```python
from build123d import *

# Parameters (mm, degrees)
BOSS_EXTRUDE1_DEPTH     = 114.3
CUT_EXTRUDE1_DEPTH      = 116.702506455
CUT_EXTRUDE1_DEPTH_BACK = 116.702506455
SKETCH5_R               = 0.55245


with BuildPart() as part:
    # Sketch4 → Boss-Extrude1 (new, symmetric)
    with BuildSketch(Plane.XY):
        with BuildLine():
            Line((4.190365, -12.7), (10.11729625, -12.7))
            ThreePointArc((10.11729625, -12.7), (11.943543585, -11.943543585), (12.7, -10.11729625))
            Line((12.7, -10.11729625), (12.7, -4.190365))
            ThreePointArc((12.7, -4.190365), (12.42492494, -3.52627506), (11.760835, -3.2512))
            Line((11.760835, -3.2512), (11.429365, -3.2512))
            ThreePointArc((11.429365, -3.2512), (10.76527506, -3.52627506), (10.4902, -4.190365))
            Line((10.4902, -4.190365), (10.4902, -6.348478019))
            ThreePointArc((10.4902, -6.348478019), (9.830707141, -7.335478831), (8.666460301, -7.103895736))
            Line((8.666460301, -7.103895736), (5.299899128, -3.737334563))
            ThreePointArc((5.299899128, -3.737334563), (4.817571085, -3.015479634), (4.6482, -2.16399369))
            Line((4.6482, -2.16399369), (4.6482, 0))
            Line((4.6482, 0), (2.6035, 0))
            ThreePointArc((2.6035, 0), (1.840952505, -1.840952505), (0, -2.6035))
            Line((0, -2.6035), (0, -4.6482))
            Line((0, -4.6482), (2.16399369, -4.6482))
            ThreePointArc((2.16399369, -4.6482), (3.015479634, -4.817571085), (3.737334563, -5.299899128))
            Line((3.737334563, -5.299899128), (7.103895736, -8.666460301))
            ThreePointArc((7.103895736, -8.666460301), (7.335478831, -9.830707141), (6.348478019, -10.4902))
            Line((6.348478019, -10.4902), (4.190365, -10.4902))
            ThreePointArc((4.190365, -10.4902), (3.52627506, -10.76527506), (3.2512, -11.429365))
            Line((3.2512, -11.429365), (3.2512, -11.760835))
            ThreePointArc((3.2512, -11.760835), (3.52627506, -12.42492494), (4.190365, -12.7))
        make_face()
    extrude(amount=BOSS_EXTRUDE1_DEPTH, both=True)

    # Sketch5 → Cut-Extrude1 (cut, two sides: drawn at the far end of the back side and taken through both)
    with BuildSketch(Plane.XY.offset(-CUT_EXTRUDE1_DEPTH_BACK)):
        with Locations((10.356153152, -12.7)):
            Circle(SKETCH5_R)
        with Locations((5.796028019, -12.7)):
            Circle(SKETCH5_R)
        with Locations((12.7, -10.356153152)):
            Circle(SKETCH5_R)
        with Locations((12.7, -5.796028019)):
            Circle(SKETCH5_R)
    extrude(amount=CUT_EXTRUDE1_DEPTH + CUT_EXTRUDE1_DEPTH_BACK, mode=Mode.SUBTRACT)

    # Mirror1: part across plane


with BuildPart() as part_1:
    add(part.part)
    add(part.part.mirror(Plane(origin=(0, 0, 0), x_dir=(0, 0, 1), z_dir=(1, 0, 0))))

    # Mirror2: part across plane


with BuildPart() as part_2:
    add(part_1.part)
    add(part_1.part.mirror(Plane.ZX))


solid = part_2.part
```
The listing builds one solid part. Answer for the finished solid, in the listing's coordinates (mm). A direction names the side the tool comes from. Round coordinates to 2 decimals unless told otherwise and drop trailing zeros. Put each result on its own line as item: value. Start each with the question number.
(1) Given P1, Ø5, axis at y = -0.5, z = 48.5, coming from the -X side; P2, Ø3.5, axis at x = 0, z = -49.5, coming from the +Y side; P3, Ø1, axis at y = 2, z = -50.5, coming from the +X side, each flat-ended and moving along its own axis, determine where each tip first touches the part or whether it passes through.
(2) Straight lines are drawn through the part: probe 1 along Y at (x, z) = (-5.5, 15.5); probe 2 along X at (y, z) = (-6.25, -45.5); probe 3 along Y at (x, z) = (0, 27). For each, find the intervals that lie inside material, in ascending order. Write a range as from..to.
(3) For faces 5 (the flat face through (4.648, 0, 2)), 6 (the flat face through (0, -3, -114.3)), determine the directions among +Z, -Z, +X, -X, +Y, -Y from which every point of the face is accessible in a straight line to the end or side of a thin tool.
(4) Determine the mould class of faces 1 (the flat face through (0, -4.648, 2)), 2 (the flat face through (-4.648, 0, 2)), 3 (the flat face through (0, 4.648, 2)), 4 (the flat face through (0, -3, 114.3)) for opening direction Y: released by +Y, released by -Y, zero draft, split by the parting line, or undercut.
Reply:
1. P1: x = -4.81
1. P2: y = 4.65
1. P3: x = 4.67
2. probe 1: -12.23..-10.49, -7.06..-3.94, 3.94..7.06, 10.49..12.23
2. probe 2: -12.39..-10.49, -7.81..-4.69, 4.69..7.81, 10.49..12.39
2. probe 3: -4.65..-2.6, 2.6..4.65
3. face 5: +Z, -Z, +X
3. face 6: -Z, +X, -X, +Y, -Y
4. face 1: released by -Y
4. face 2: undercut
4. face 3: released by +Y
4. face 4: zero draft
